Verification items for the finished model (mm, model axes). Coordinates: 2 decimals unless noted, no trailing zeros. Order: outer loops, then holes, each group sorted by start corner. A loop starts at its lowest first (then second) coordinate and runs counter-clockwise, first axis right, second up. Notation, with made-up numbers: (79, 75.5) -> (102, 75.5) arc R27 ccw to (102, 113.5) -> close; hole circle Ø7 at (23, 62). An arc over 180 degrees is marked (long way). Use CSV: the item, a comma, the result in double quotes. Start each with the question number.
1) Sectioned sample at C-C on z = 0.35. Record the boundary of the cut face in (x, y) (3 decimals), then the cut area to 3 significant figures.
2) Sectioned sample at B-B on y = 10.5. Record the boundary of the cut face in (x, z), then the cut area to 3 significant figures.
3) Sectioned sample at A-A on x = 28.99. Record the boundary of the cut face in (y, z).
4) Scan lines: line 1 along X through (y, z) = (6.25, 0.45); line 2 along Y through (x, z) = (4, 0.5); line 3 along Y through (x, z) = (12, 0.2) (3 decimals). Record each from-to range of solid material in increasing order.
from build123d import *

# Parameters (mm, degrees)
SKETCH1_R           = 1.6002
BOSS_EXTRUDE1_DEPTH = 0.7874


with BuildPart() as part:
    # Sketch1 → Boss-Extrude1 (new body)
    with BuildSketch(Plane.XY):
        with BuildLine():
            Line((1.27, 0), (31.72, 0))
            ThreePointArc((31.72, 0), (32.618025612, 0.371974388), (32.99, 1.27))
            Line((32.99, 1.27), (32.99, 13.74))
            ThreePointArc((32.99, 13.74), (32.618025612, 14.638025612), (31.72, 15.01))
            Line((31.72, 15.01), (1.27, 15.01))
            ThreePointArc((1.27, 15.01), (0.371974388, 14.638025612), (0, 13.74))
            Line((0, 13.74), (0, 1.27))
            ThreePointArc((0, 1.27), (0.371974388, 0.371974388), (1.27, 0))
        make_face()
        with Locations((4, 7.505)):
            Circle(SKETCH1_R, mode=Mode.SUBTRACT)
        with Locations((28.99, 7.505)):
            Circle(SKETCH1_R, mode=Mode.SUBTRACT)
        with BuildLine():
            Line((11.02246495, 12.305), (21.96753505, 12.305))
            ThreePointArc((21.96753505, 12.305), (24.302438512, 11.216216634), (24.969229081, 8.727720354))
            Line((24.969229081, 8.727720354), (24.351379341, 5.223720354))
            ThreePointArc((24.351379341, 5.223720354), (23.308901944, 3.418096537), (21.349685309, 2.705))
            Line((21.349685309, 2.705), (11.640314691, 2.705))
            ThreePointArc((11.640314691, 2.705), (9.681098056, 3.418096537), (8.638620659, 5.223720354))
            Line((8.638620659, 5.223720354), (8.020770919, 8.727720354))
            ThreePointArc((8.020770919, 8.727720354), (8.687561488, 11.216216634), (11.02246495, 12.305))
        make_face(mode=Mode.SUBTRACT)
    extrude(amount=BOSS_EXTRUDE1_DEPTH)


solid = part.part
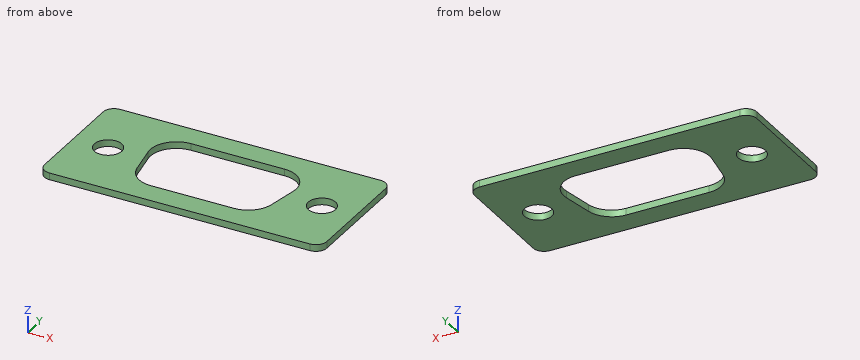
Answers follow:
1,outline,"(0, 1.27) arc R1.27 ccw to (1.27, 0) -> (31.72, 0) arc R1.27 ccw to (32.99, 1.27) -> (32.99, 13.74) arc R1.27 ccw to (31.72, 15.01) -> (1.27, 15.01) arc R1.27 ccw to (0, 13.74) -> close; hole circle Ø3.2 at (4, 7.505); hole (8.021, 8.728) -> (8.639, 5.224) arc R3.048 ccw to (11.64, 2.705) -> (21.35, 2.705) arc R3.048 ccw to (24.351, 5.224) -> (24.969, 8.728) arc R3.048 ccw to (21.968, 12.305) -> (11.022, 12.305) arc R3.048 ccw to start; hole circle Ø3.2 at (28.99, 7.505)"
1,area,"328 mm²"
2,outline,"(0, 0) -> (8.24, 0) -> (8.24, 0.79) -> (0, 0.79) -> close; (24.75, 0) -> (32.99, 0) -> (32.99, 0.79) -> (24.75, 0.79) -> close"
2,area,"13.0 mm²"
3,outline,"(0, 0) -> (5.9, 0) -> (5.9, 0.79) -> (0, 0.79) -> close; (9.11, 0) -> (15.01, 0) -> (15.01, 0.79) -> (9.11, 0.79) -> close"
4,line 1,"x = 0 to 3.01, 4.99 to 8.46, 24.53 to 28, 29.98 to 32.99"
4,line 2,"y = 0 to 5.9, 9.11 to 15.01"
4,line 3,"y = 0 to 2.705, 12.305 to 15.01"
